Autodesk Inventor part; units mm, degrees
ref_plane "Work Plane2" through (-89, -40.3889, 33.5) normal (0, 0, 1) x (1, 0, 0)
ref_plane "YZ Plane" through (0, 0, 0) normal (1, 0, 0) x (0, 1, 0)
ref_plane "XZ Plane" through (0, 0, 0) normal (0, 1, 0) x (-1, 0, 0)
ref_plane "Work Plane1" through (0, 0, 0) normal (0, 0, 1) x (1, 0, 0)
sketch "Sketch1" plane through (0, 0, 0) normal (0, 0, 1) x (1, 0, 0)
  line L0 (23.5, 88.5) -> (-23.5, 88.5)
  line L1 (-23.5, 88.5) -> (-23.5, 36.5)
  line L2 (-26.5, 33.5) -> (-89, 33.5)
  line L3 (-89, 33.5) -> (-89, -72.5)
  line L4 (-89, -72.5) -> (-77, -72.5)
  line L5 (-74, -75.5) -> (-74, -93.5)
  line L6 (-74, -93.5) -> (74, -93.5)
  line L7 (74, -93.5) -> (74, -75.5)
  line L8 (77, -72.5) -> (89, -72.5)
  line L9 (89, -72.5) -> (89, 33.5)
  line L10 (89, 33.5) -> (26.5, 33.5)
  line L11 (23.5, 36.5) -> (23.5, 88.5)
  line L12 (-4.5, 81.5) -> (-4.5, 36.5)
  line L13 (-7.5, 33.5) -> (-13.5, 33.5)
  line L14 (-16.5, 36.5) -> (-16.5, 81.5)
  line L15 (-13.5, 84.5) -> (-7.5, 84.5)
  line L16 (16.5, 81.5) -> (16.5, 36.5)
  line L17 (13.5, 33.5) -> (7.5, 33.5)
  line L18 (4.5, 36.5) -> (4.5, 81.5)
  line L19 (7.5, 84.5) -> (13.5, 84.5)
  line L20 (-16.5, 88.5) -> (-22.5, 88.5)
  line L21 (-22.5, 88.5) -> (-22.5, 3.75)
  line L22 (-22.5, 3.75) -> (-16.5, 3.75)
  line L23 (-16.5, 3.75) -> (-16.5, 88.5)
  line L24 (-32.2, 4.75) -> (-59.9, 4.75)
  arc A0 (13.5, 33.5) -> (16.5, 36.5) centre (13.5, 36.5) ccw
  arc A1 (4.5, 36.5) -> (7.5, 33.5) centre (7.5, 36.5) ccw
  arc A2 (7.5, 84.5) -> (4.5, 81.5) centre (7.5, 81.5) ccw
  arc A3 (16.5, 81.5) -> (13.5, 84.5) centre (13.5, 81.5) ccw
  arc A4 (-4.5, 81.5) -> (-7.5, 84.5) centre (-7.5, 81.5) ccw
  arc A5 (-7.5, 33.5) -> (-4.5, 36.5) centre (-7.5, 36.5) ccw
  arc A6 (-16.5, 36.5) -> (-13.5, 33.5) centre (-13.5, 36.5) ccw
  arc A7 (-13.5, 84.5) -> (-16.5, 81.5) centre (-13.5, 81.5) ccw
  arc A8 (-26.5, 33.5) -> (-23.5, 36.5) centre (-26.5, 36.5) ccw
  arc A9 (-74, -75.5) -> (-77, -72.5) centre (-77, -75.5) ccw
  arc A10 (77, -72.5) -> (74, -75.5) centre (77, -75.5) ccw
  arc A11 (23.5, 36.5) -> (26.5, 33.5) centre (26.5, 36.5) ccw
  point P0 (0, 0)
  point P1 (-16.5, 36.5)
  point P2 (-16.5, 81.5)
  dimension "d0" = 1
  dimension "d2" = 1
ref_plane "Work Plane2" through (-89, -40.3889, 33.5) normal (0, 0, 1) x (1, 0, 0)
extrude "Extrusion1" add sketch "Sketch1" along normal up to surface (33.5 mm away) contours L23 L14 L22 L21 L0
sketch "Sketch2" plane through (-22.5, 3.75, 0) normal (-1, 0, 0) x (0, 0, 1)
  arc A0 (15.7043, 9.7757) -> (16.863, 11.545) centre (12.3771, 13.2188) ccw
  arc A1 (16.863, 11.545) -> (17.4685, 11.512) centre (17.375, 15.375) ccw
  arc A2 (17.4685, 11.512) -> (18.4285, 9.6275) centre (22.1095, 12.6893) ccw
  arc A3 (18.4285, 9.6275) -> (19.3146, 9.863) centre (17.375, 15.375) ccw
  arc A4 (19.3146, 9.863) -> (19.2121, 11.9755) centre (14.599, 10.6929) ccw
  arc A5 (19.2121, 11.9755) -> (19.7212, 12.3047) centre (17.375, 15.375) ccw
  arc A6 (19.7212, 12.3047) -> (21.6056, 11.3444) centre (22.7839, 15.9851) ccw
  arc A7 (21.6056, 11.3444) -> (22.184, 12.0558) centre (17.375, 15.375) ccw
  arc A8 (22.184, 12.0558) -> (20.8594, 13.7045) centre (17.8813, 9.9554) ccw
  arc A9 (20.8594, 13.7045) -> (21.0778, 14.2702) centre (17.375, 15.375) ccw
  arc A10 (21.0778, 14.2702) -> (23.1668, 14.6008) centre (21.3923, 19.0479) ccw
  arc A11 (23.1668, 14.6008) -> (23.2166, 15.5164) centre (17.375, 15.375) ccw
  arc A12 (23.2166, 15.5164) -> (21.1758, 16.0716) centre (20.9701, 11.288) ccw
  arc A13 (21.1758, 16.0716) -> (21.02, 16.6576) centre (17.375, 15.375) ccw
  arc A14 (21.02, 16.6576) -> (22.5157, 18.153) centre (18.4662, 20.7077) ccw
  arc A15 (22.5157, 18.153) -> (22.0178, 18.923) centre (17.375, 15.375) ccw
  arc A16 (22.0178, 18.923) -> (20.0404, 18.1726) centre (22.6858, 14.1817) ccw
  arc A17 (20.0404, 18.1726) -> (19.57, 18.5552) centre (17.375, 15.375) ccw
  arc A18 (19.57, 18.5552) -> (19.9011, 20.644) centre (15.1233, 20.3306) ccw
  arc A19 (19.9011, 20.644) -> (19.0457, 20.9743) centre (17.375, 15.375) ccw
  arc A20 (19.0457, 20.9743) -> (17.887, 19.205) centre (22.3729, 17.5312) ccw
  arc A21 (17.887, 19.205) -> (17.2815, 19.238) centre (17.375, 15.375) ccw
  arc A22 (17.2815, 19.238) -> (16.3215, 21.1225) centre (12.6405, 18.0607) ccw
  arc A23 (16.3215, 21.1225) -> (15.4354, 20.887) centre (17.375, 15.375) ccw
  arc A24 (15.4354, 20.887) -> (15.5379, 18.7745) centre (20.151, 20.0571) ccw
  arc A25 (15.5379, 18.7745) -> (15.0288, 18.4453) centre (17.375, 15.375) ccw
  arc A26 (15.0288, 18.4453) -> (13.1444, 19.4056) centre (11.9661, 14.7649) ccw
  arc A27 (13.1444, 19.4056) -> (12.566, 18.6942) centre (17.375, 15.375) ccw
  arc A28 (12.566, 18.6942) -> (13.8906, 17.0455) centre (16.8687, 20.7946) ccw
  arc A29 (13.8906, 17.0455) -> (13.6722, 16.4798) centre (17.375, 15.375) ccw
  arc A30 (13.6722, 16.4798) -> (11.5832, 16.1492) centre (13.3577, 11.7021) ccw
  arc A31 (11.5832, 16.1492) -> (11.5334, 15.2336) centre (17.375, 15.375) ccw
  arc A32 (11.5334, 15.2336) -> (13.5742, 14.6784) centre (13.7799, 19.462) ccw
  arc A33 (13.5742, 14.6784) -> (13.73, 14.0924) centre (17.375, 15.375) ccw
  arc A34 (13.73, 14.0924) -> (12.2343, 12.597) centre (16.2838, 10.0423) ccw
  arc A35 (12.2343, 12.597) -> (12.7322, 11.827) centre (17.375, 15.375) ccw
  arc A36 (12.7322, 11.827) -> (14.7096, 12.5774) centre (12.0642, 16.5683) ccw
  arc A37 (14.7096, 12.5774) -> (15.18, 12.1948) centre (17.375, 15.375) ccw
  arc A38 (15.18, 12.1948) -> (14.8489, 10.106) centre (19.6267, 10.4194) ccw
  arc A39 (14.8489, 10.106) -> (15.7043, 9.7757) centre (17.375, 15.375) ccw
  circle A40 centre (17.375, 15.375) radius 6.75
  circle A41 centre (17.375, 15.375) radius 5.8433
  line L0 (23.2183, 15.375) -> (24.125, 15.375)
  circle A42 centre (10.5, 57.25) radius 5.5
  point P0 (0, -3.75)
  dimension "d6" = 13.5
  dimension "d5" = 0.9067
  dimension "d9" = 11
extrude "Extrusion2" cut sketch "Sketch2" against normal up to next contours A39 A38 A37 A36 A35 A34 A33 A32 A31 A30 A29 A28 A27 A26 A25 A24 A23 A22 A21 A20 A19 A18 A17 A16 A15 A14 A13 A12 A11 A10 A9 A8 A7 A6 A5 A4 A3 A2 A1 A0 | A0 A1 A2 A41 | A41 A36 A37 A38 | A4 A5 A6 A41 | A41 A32 A33 A34 | A8 A9 A10 A41 | A41 A28 A29 A30 | A41 A24 A25 A26 | A12 A13 A14 A41 | A41 A20 A21 A22 | A16 A17 A18 A41 | A40 | A42
sketch "Sketch3" plane through (-16.5, 3.75, 0) normal (1, 0, 0) x (0, 0, -1)
  circle A0 centre (-23.4363, 30.1825) radius 2
  point P0 (0, -3.75)
extrude "Extrusion3" cut sketch "Sketch3" against normal blind 5
ref_plane "Work Plane3" through (-23.5, 3.75, 0) normal (-1, 0, 0) x (0, 0, 1)
sketch "Sketch5" plane through (-23.5, 3.75, 0) normal (-1, 0, 0) x (0, 0, 1)
  circle A0 centre (29.5, 80.75) radius 2.1
  circle A1 centre (4, 80.75) radius 2.1
  circle A2 centre (3.5, 33.25) radius 2.1
  point P0 (0, -3.75)
hole "Hole1" at (-23.5, 84.5, 29.5) at (-23.5, 84.5, 4) at (-23.5, 37, 3.5) direction (1, 0, 0) diameter 3.6 end through all countersink diameter 6.2 countersink angle 90
sketch "Sketch6" plane through (-22.5, 3.75, 33.5) normal (0, 0, 1) x (1, 0, 0)
  line L0 (0, 8.625) -> (0, 22.125)
  line L1 (1, 32.1825) -> (1, 28.1825)
  line L2 (0, 31.15) -> (0, 35.35)
  line L3 (0, 51.75) -> (0, 62.75)
  line L4 (0, 78.65) -> (0, 82.85)
  line L5 (0, 78.65) -> (0, 82.85)
  line L6 (6, 0) -> (0, 0)
  line L7 (6, 84.75) -> (6, 0)
  line L8 (0, 84.75) -> (6, 84.75)
  line L9 (0, 0) -> (0, 84.75)
  line L10 (6, 28.125) -> (0, 28.125)
  line L11 (0, 28.125) -> (0, 35.35)
  line L12 (0, 35.35) -> (6, 35.35)
  line L13 (6, 35.35) -> (6, 28.125)
  line L14 (0, 8.625) -> (6, 8.625)
  line L15 (6, 8.625) -> (0, 8.625)
  line L16 (0, 8.625) -> (0, 22.125)
  line L17 (0, 22.125) -> (6, 22.125)
  line L18 (6, 22.125) -> (6, 8.625)
  line L19 (6, 78.95) -> (0.3, 78.95)
  line L20 (6, 84.75) -> (0, 84.75)
  line L21 (6, 78.95) -> (0, 78.95)
  line L22 (0, 78.95) -> (0, 84.75)
  line L23 (0, 84.75) -> (6, 84.75)
  line L24 (6, 84.75) -> (6, 78.95)
  line L25 (0, 51.75) -> (6, 51.75)
  line L26 (0, 51.75) -> (0, 62.75)
  line L27 (6, 51.75) -> (0, 51.75)
  line L28 (0, 51.75) -> (0, 62.75)
  line L29 (0, 62.75) -> (6, 62.75)
  line L30 (6, 62.75) -> (6, 51.75)
  line L31 (6, 0) -> (0, 0)
  line L32 (0, 0) -> (0, 4)
  line L33 (0, 4) -> (6, 4)
  line L34 (6, 4) -> (6, 0)
  circle A0 centre (3, 5.8) radius 1.8
  line L35 (6, 22.125) -> (0, 28.125)
  line L36 (0, 22.125) -> (6, 28.125)
  line L37 (6, 35.35) -> (0, 51.75)
  line L38 (0, 35.35) -> (6, 51.75)
  line L39 (0.3, 82.55) -> (0.3, 78.95)
  line L40 (6, 62.75) -> (0.3, 78.95)
  line L41 (6, 82.55) -> (6, 78.95)
  line L42 (0.3, 78.95) -> (6, 78.95)
  line L43 (6, 78.95) -> (0, 62.75)
  point P0 (22.5, -3.75)
  point P1 (3, 25.125)
  point P2 (3.0769, 71.0577)
  point P3 (3, 43.55)
  dimension "d20" = 4
  dimension "d21" = 3.6
  dimension "d22" = 3
  dimension "d23" = 3
hole "Hole2" at (-19.5, 28.875, 33.5) at (-19.5, 9.55, 33.5) at (-19.4231, 74.8077, 33.5) at (-19.5, 47.3, 33.5) direction (0, 0, -1) diameter 3.6 end through all countersink diameter 6.3 countersink angle 90
sketch "Sketch9" plane through (-22.5, 88.5, 0) normal (0, 1, 0) x (1, 0, 0)
  circle A0 centre (22.5, -20.825) radius 2.3
  circle A1 centre (22.5, -12.675) radius 2.3
  line L0 (18, -33.5) -> (27, -33.5)
  line L1 (27, 0) -> (27, -33.5)
  line L2 (27, 0) -> (18, 0)
  line L3 (18, 0) -> (18, -33.5)
  line L4 (22.5, -20.825) -> (0, -20.825)
  line L5 (0, -24.125) -> (0, -10.625)
  line L6 (22.5, -12.675) -> (0, -12.675)
  line L7 (6, 0) -> (6, -33.5)
  point P0 (22.5, 0)
  point P1 (3, -20.825)
  point P2 (3, -12.675)
  dimension "d45" = 3
  dimension "d46" = 3
  dimension "d47" = 3
  dimension "d48" = 3
hole "Hole5" at (-19.5, 88.5, 20.825) at (-19.5, 88.5, 12.675) direction (0, -1, 0) diameter 4 depth 6 counterbore diameter 4.6 counterbore depth 1.5
sketch "Sketch10" plane through (-19.5, 47.3, 33.5) normal (0, 0, 1) x (1, 0, 0)
  line L0 (-3, 8.2) -> (-3, 19.2)
  arc A0 (3, -17.4645) -> (-3, -17.4645) centre (0, -18.425) ccw
  arc A1 (-3, -0.9605) -> (3, -0.9605) centre (0, 0) ccw
  arc A2 (3, -17.4645) -> (-3, -17.4645) centre (0, -18.425) ccw
  line L1 (3, -0.9605) -> (3, -17.4645)
  arc A3 (-3, -0.9605) -> (3, -0.9605) centre (0, 0) ccw
  line L2 (-3, -17.4645) -> (-3, -0.9605)
  line L3 (3, 8.2) -> (-3, 8.2)
  line L4 (3, 19.2) -> (-3, 19.2)
  line L5 (-3, 19.2) -> (3, 8.2)
  line L6 (-3, 8.2) -> (3, 19.2)
  line L7 (3, -17.4645) -> (-3, -0.9605)
  line L8 (-3, -17.4645) -> (3, -0.9605)
  point P0 (19.5, -47.3)
  point P1 (0, -9.2125)
  point P2 (0, 13.7)
hole "Hole6" at (-19.5, 38.0875, 33.5) at (-19.5, 61, 33.5) direction (0, 0, -1) diameter 4 depth 6 counterbore diameter 4.6 counterbore depth 1.5
sketch "Sketch11" plane through (-22.5, 3.75, 0) normal (0, -1, 0) x (1, 0, 0)
  line L0 (6, 33.5) -> (0, 33.5)
  line L1 (0, 0) -> (0, 33.5)
  line L2 (0, 0) -> (6, 0)
  line L3 (6, 0) -> (6, 33.5)
  point P0 (22.5, 0)
extrude "Extrusion4" cut sketch "Sketch11" against normal blind 2
equation "\"d22\" = d23"
properties part number "right_gear_holder"
Geometry: final body of the model. Coordinates: model frame, mm. A direction names the side the tool comes from. Give positions to 0.01 mm unless a question says otherwise; leave off trailing zeros. Order: outer loops, then holes, each group sorted by start corner. A loop starts at its lowest first (then second) coordinate and runs counter-clockwise, first axis right, second up. Notation, with made-up numbers: (25.25, 84.5) -> (50.25, 84.5) arc R12 cw to (50.25, 90.5) -> close; hole circle Ø5 at (72, 45). An arc over 180 degrees is marked (long way). Answer as a JSON object with one key per item and string values.
Q1. Section B-B (z = 9). State how many separate pieces and enclosed holes the cut face has, plus the area to 3 significant figures.
Entries:
{"separate pieces": "2", "enclosed holes": "4", "area": "392 mm^2"}
Q2. Section A-A (y = 84.5). Output: boundary loops of the cut face in (x, z) (3 decimals).
Entries:
{"outline": "(-22.5, 0) -> (-16.5, 0) -> (-16.5, 2.2) -> (-22.2, 2.2) -> (-22.5, 1.9) -> close; (-22.5, 6.1) -> (-22.2, 5.8) -> (-16.5, 5.8) -> (-16.5, 27.7) -> (-22.2, 27.7) -> (-22.5, 27.4) -> close; (-22.5, 31.6) -> (-22.2, 31.3) -> (-16.5, 31.3) -> (-16.5, 33.5) -> (-22.5, 33.5) -> close; hole circle Ø4 at (-19.5, 12.675); hole circle Ø4 at (-19.5, 20.825)"}
Q3. Material intervals for probe 1 along Z at (x, y) = (-19.5, 87.75) (3 decimals); probe 2 along Y at (x, z) = (-19, 27); probe 3 along X at (y, z) = (47.5, 31), sorted ascending.
Entries:
{"probe 1": "z = 0 to 10.375, 14.975 to 18.525, 23.125 to 33.5", "probe 2": "y = 5.75 to 7.82, 11.28 to 27.15, 30.6 to 45.57, 49.03 to 73.06, 76.56 to 88.5", "probe 3": "x = -22.5 to -21.29, -17.71 to -16.5"}
Q4. First-contact query: pin 1 (10 mm diameter, centred on y = 61, z = 10.5, fed in from +X); pin 2 (15.5 mm diameter, centred on y = 19.125, z = 17.375, fed in from -X); pin 3 (3 mm diameter, centred on x = -19.5, z = 20.825, fed in from +Y). Flat tips, straight axial feed; report the tip coordinate or a pass-through.
Entries:
{"pin 1": "passes through", "pin 2": "stops at x = -22.5", "pin 3": "stops at y = 82.5"}
Q5. Section C-C (y = 61). Output: boundary loops of the cut face in (x, z).
Entries:
{"outline": "(-22.5, 0) -> (-16.5, 0) -> (-16.5, 5) -> (-22.5, 5) -> close; (-22.5, 16) -> (-16.5, 16) -> (-16.5, 33.5) -> (-17.2, 33.5) -> (-17.2, 32) -> (-17.5, 32) -> (-17.5, 27.5) -> (-21.5, 27.5) -> (-21.5, 32) -> (-21.8, 32) -> (-21.8, 33.5) -> (-22.5, 33.5) -> close"}
Q6. Draft query along Y for faces 4 (the flat face through (-16.5, 47, 17)), 5 (the flat face through (-20, 61, 27.5)), 6 (the flat face through (-19, 88.5, 17)). Return one class per face: released by +Y, released by -Y, zero draft, split by the parting line, or undercut.
Entries:
{"face 4": "zero draft", "face 5": "undercut", "face 6": "released by +Y"}
Q7. Access query for faces 1 (the cylindrical face through (-21.483, 61.26, 29.718)), 2 (the flat face through (-20, 82.5, 13)), 3 (the cylindrical face through (-20.04, 27.16, 15.85)). Directions: +Z, -Z, +X, -X, +Y, -Y. A direction counts if a zero-diameter tool reaches every point of the face in a straight line with its end or side. Return the directions, or none.
Entries:
{"face 1": "+Z", "face 2": "+Y", "face 3": "+Z, -Z"}
